Check sheet for the modelled part. Datum: model origin and axes. Units: mm. A direction names the side the tool comes from. Round coordinates to 2 decimals unless told otherwise and drop trailing zeros. Loops run counter-clockwise (first coordinate to the right, second up) from the corner with the lowest first, then second, coordinate; pieces in that order, holes last. Notation, with made-up numbers: (-14.5, -6.75) -> (39.5, -6.75) arc R17 ccw to (39.5, 20.25) -> close; hole circle Ø6 at (2, 18.25). An arc over 180 degrees is marked (long way). Use one line per item in the form item = value. Start each with the question number.
(1) Set-up check for faces 4 (the flat face through (-50, -20, 20)), 5 (the flat face through (0, -25, 30)): record each of +Z, -Z, +X, -X, +Y, -Y from which the full face is reachable in a straight line by a thin tool's end or side.
(2) Sectioned sample at D-D (z = 3). Record the cut outline in (x, y), and give its area (3 significant figures).
(3) Material ranges on probe 1 along X at (y, z) = (-7, 22) (3 decimals); probe 2 along X at (y, z) = (-30, 28); probe 3 along Z at (x, y) = (31, -14), recorded low to high. Write a range as [from, to].
(4) Go/stop test with flat-tipped pins: pin 1 (1 mm diameter, centred on x = 12, z = 19, fed in from +Y); pin 2 (3 mm diameter, centred on x = -1, z = 24, fed in from +Y); pin 3 (16 mm diameter, centred on x = 0, z = 30, fed in from +Y). Record where each tip stops, or that it passes through.
(5) Sectioned sample at C-C (y = -27). Record the cut outline in (x, z), and give its area (3 significant figures).
(6) Sectioned sample at A-A (z = 20). Record the cut outline in (x, y).
(7) Sectioned sample at B-B (x = -35). Record the cut outline in (y, z).
(8) Draft check along Z on faces 1 (the cylindrical face through (0, -32, 35)), 2 (the cylindrical face through (49.43, -19.75, 39.4)), 3 (the cylindrical face through (20.576, -0.509, 20.252)). Enter one of: released by +Z, released by -Z, zero draft, split by the parting line, or undercut.
from build123d import *

# Parameters (mm, degrees)
DODANIE_WYCI_GNI_CIE1_DEPTH = 40
WYTNIJ_WYCI_GNI_CIE3_REACH  = 77.498
SZKIC2_R                    = 6.5
SZKIC3_R                    = 5
WYTNIJ_WYCI_GNI_CIE6_DEPTH  = 15
SFAZOWANIE1_SIZE            = 2
ZAOKR_GLENIE1_R             = 2


with BuildPart() as part:
    # Szkic1 → Dodanie-wyciągnięcie1 (new body)
    with BuildSketch(Plane.XY):
        with BuildLine():
            Line((50, 0), (20, 0))
            ThreePointArc((20, 0), (0, -20), (-20, 0))
            Line((-20, 0), (-50, 0))
            Line((-50, 0), (-50, -40))
            Line((-50, -40), (50, -40))
            Line((50, -40), (50, 0))
        make_face()
    extrude(amount=DODANIE_WYCI_GNI_CIE1_DEPTH)

    # Szkic2 → Wytnij-wyciągnięcie3 (cut, up to next)
    with BuildSketch(Plane(origin=(0, 0, 0), x_dir=(1, 0, 0), z_dir=(0, 1, 0)), mode=Mode.PRIVATE) as wytnij_wyci_gni_cie3_sk1:
        with Locations(Location((-35, -20, 0), (0, 0, 270))):
            Circle(SZKIC2_R)
    wytnij_wyci_gni_cie3_tool1 = extrude(wytnij_wyci_gni_cie3_sk1.sketch, amount=-WYTNIJ_WYCI_GNI_CIE3_REACH, mode=Mode.PRIVATE) & part.part
    # Szkic2 → Wytnij-wyciągnięcie3 (cut, up to next)
    with BuildSketch(Plane(origin=(0, 0, 0), x_dir=(1, 0, 0), z_dir=(0, 1, 0)), mode=Mode.PRIVATE) as wytnij_wyci_gni_cie3_sk2:
        with Locations(Location((35, -20, 0), (0, 0, 270))):
            Circle(SZKIC2_R)
    wytnij_wyci_gni_cie3_tool2 = extrude(wytnij_wyci_gni_cie3_sk2.sketch, amount=-WYTNIJ_WYCI_GNI_CIE3_REACH, mode=Mode.PRIVATE) & part.part
    add(wytnij_wyci_gni_cie3_tool1.solids().sort_by_distance((-35, 0, 20))[0], mode=Mode.SUBTRACT)
    add(wytnij_wyci_gni_cie3_tool2.solids().sort_by_distance((35, 0, 20))[0], mode=Mode.SUBTRACT)

    # Szkic3 → Wytnij-wyciągnięcie6 (cut)
    with BuildSketch(Plane(origin=(0, -40, 0), x_dir=(-1, 0, 0), z_dir=(0, -1, 0))):
        with Locations(Location((0, -30, 0), (0, 0, 90))):
            Circle(SZKIC3_R)
    extrude(amount=-WYTNIJ_WYCI_GNI_CIE6_DEPTH, mode=Mode.SUBTRACT)

    # Sfazowanie1
    sfazowanie1_edges = [part.edges().sort_by_distance(p)[0] for p in [
        (-35, 0, 13.5),
        (-35, -40, 13.5),
        (35, 0, 13.5),
        (35, -40, 13.5),
        (0, -40, 35),
    ]]
    chamfer(sfazowanie1_edges, length=SFAZOWANIE1_SIZE)

    # Zaokrąglenie1
    zaokr_glenie1_edges = [part.edges().sort_by_distance(p)[0] for p in [
        (0, -20, 0),
        (-35, 0, 40),
        (20, 0, 20),
        (50, 0, 20),
        (50, -40, 20),
        (-50, -40, 20),
        (-50, 0, 20),
        (-20, 0, 20),
        (-50, -20, 40),
        (0, -40, 40),
        (50, -20, 40),
        (35, 0, 40),
        (0, -20, 40),
        (35, 0, 0),
        (50, -20, 0),
        (0, -40, 0),
        (-50, -20, 0),
        (-35, 0, 0),
    ]]
    fillet(zaokr_glenie1_edges, radius=ZAOKR_GLENIE1_R)


solid = part.part
Checks:
q1.face_4 = +Z, -Z, -X, +Y, -Y
q1.face_5 = -Y
q2.outline = (-50, -38) arc R2 ccw to (-48, -40) -> (48, -40) arc R2 ccw to (50, -38) -> (50, -2) arc R2 ccw to (48, 0) -> (21.91, 0) arc R2 ccw to (19.92, -1.82) arc R20 cw to (-19.92, -1.82) arc R2 ccw to (-21.91, 0) -> (-48, 0) arc R2 ccw to (-50, -2) -> close
q2.area = 3,370 mm2
q3.probe_1 = [-50, -41.185], [-28.815, -18.735], [18.735, 28.815], [41.185, 50]
q3.probe_2 = [-50, -4.58], [4.58, 50]
q3.probe_3 = [0, 14.88], [25.12, 40]
q4.pin_1 = -15.61
q4.pin_2 = -19.84
q4.pin_3 = -18.33
q5.outline = (-50, 2) arc R2 ccw to (-48, 0) -> (48, 0) arc R2 ccw to (50, 2) -> (50, 38) arc R2 ccw to (48, 40) -> (-48, 40) arc R2 ccw to (-50, 38) -> close; hole circle Ø13 at (-35, 20); hole circle Ø10 at (0, 30); hole circle Ø13 at (35, 20)
q5.area = 3,650 mm2
q6.outline = (-50, -38) arc R2 ccw to (-48, -40) -> (-43.5, -40) -> (-41.5, -38) -> (-41.5, -2) -> (-43.5, 0) -> (-48, 0) arc R2 ccw to (-50, -2) -> close; (-28.5, -38) -> (-26.5, -40) -> (26.5, -40) -> (28.5, -38) -> (28.5, -2) -> (26.5, 0) -> (21.91, 0) arc R2 ccw to (19.92, -1.82) arc R20 cw to (-19.92, -1.82) arc R2 ccw to (-21.91, 0) -> (-26.5, 0) -> (-28.5, -2) -> close; (41.5, -38) -> (43.5, -40) -> (48, -40) arc R2 ccw to (50, -38) -> (50, -2) arc R2 ccw to (48, 0) -> (43.5, 0) -> (41.5, -2) -> close
q7.outline = (-40, 2) arc R2 ccw to (-38, 0) -> (-2, 0) arc R2 ccw to (0, 2) -> (0, 11.5) -> (-2, 13.5) -> (-38, 13.5) -> (-40, 11.5) -> close; (-40, 28.5) -> (-38, 26.5) -> (-2, 26.5) -> (0, 28.5) -> (0, 38) arc R2 ccw to (-2, 40) -> (-38, 40) arc R2 ccw to (-40, 38) -> close
q8.face_1 = undercut
q8.face_2 = released by +Z
q8.face_3 = zero draft
